Check sheet for the modelled part. Datum: model origin and axes. Units: mm. Face numbers are marked on the shaded views. Coordinates: 2 decimals unless noted, no trailing zeros. Loops run counter-clockwise (first coordinate to the right, second up) from the corner with the lowest first, then second, coordinate; pieces in that order, holes last. Notation, with made-up numbers: M -4,4 L 46,4 A22 cw 46,18 Z; hole C 42,6.5 d6. An arc over 180 degrees is marked long. Answer in a Markdown table with one row per item. Add a question column.
```python
from build123d import *

# Parameters (mm, degrees)
F0_W     = 20.955
F0_H     = 6.35
F1_DEPTH = 25.4
F2_R     = 1.5875
F3_R     = 1.190625
F4_DEPTH = 25.4


with BuildPart() as f1:
    # F0 (on Right) → F1 (new body)
    with BuildSketch(Plane.YZ):
        with Locations((-13.227284, 21.981973)):
            Rectangle(F0_W, F0_H)
    extrude(amount=F1_DEPTH)

    # F2
    f2_edges = [f1.edges().sort_by_distance(p)[0] for p in [
        (25.4, -13.227284, 25.156973),
        (25.4, -13.227284, 18.806973),
        (0, -13.227284, 18.806973),
        (0, -13.227284, 25.156973),
    ]]
    fillet(f2_edges, radius=F2_R)

    # F3 (on face) → F4 (cut)
    with BuildSketch(Plane(origin=(0, -2.749784, 0), x_dir=(-1, 0, 0), z_dir=(0, 1, 0))):
        with Locations((-6.35, 21.981973)):
            Circle(F3_R)
    extrude(amount=-F4_DEPTH, mode=Mode.SUBTRACT)


solid = f1.part
```
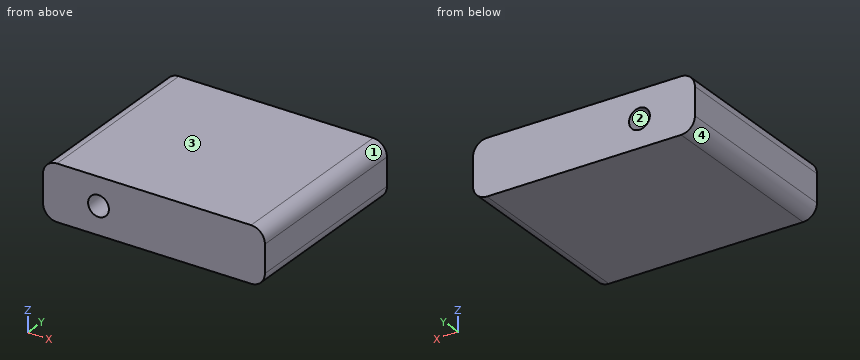
Q1. Thickness scan on L1, parallel to Z at x = 6.35, y = -9.5; L2, parallel to X at y = -16.25, z = 23; L3, parallel to X at y = -5.5, z = 22.75. Record the ranges inside material, lowest first.
Q2. Cross-section at A-A (x = 6.35). Record the cut outline in (y, z), plus the area to 3 significant figures.
Q3. Mould release check, pull along X, two halves, no side actions. Record for the marked faces 1, 2, 3 and 4: released by +X, released by -X, zero draft, split by the parting line, or undercut.
Q4. Cross-section at B-B (z = 21.5). Record the cut outline in (x, y), plus the area to 3 significant figures.
Q5. Cross-section at D-D (z = 24.5). Record the cut outline in (x, y), plus the area to 3 significant figures.
Answer key:
| question | item | result |
|---|---|---|
| 1 | L1 | 18.81 to 20.79, 23.17 to 25.16 |
| 1 | L2 | 0 to 5.73, 6.97 to 25.4 |
| 1 | L3 | 0 to 5.44, 7.26 to 25.4 |
| 2 | outline | M -23.7,18.81 L -2.75,18.81 L -2.75,20.79 L -23.7,20.79 Z; M -23.7,23.17 L -2.75,23.17 L -2.75,25.16 L -23.7,25.16 Z |
| 2 | area | 83.2 mm^2 |
| 3 | face 1 | released by +X |
| 3 | face 2 | undercut |
| 3 | face 3 | zero draft |
| 3 | face 4 | released by -X |
| 4 | outline | M 0,-23.7 L 5.26,-23.7 L 5.26,-2.75 L 0,-2.75 Z; M 7.44,-23.7 L 25.4,-23.7 L 25.4,-2.75 L 7.44,-2.75 Z |
| 4 | area | 487 mm^2 |
| 5 | outline | M 0.3,-23.7 L 25.1,-23.7 L 25.1,-2.75 L 0.3,-2.75 Z |
| 5 | area | 520 mm^2 |
